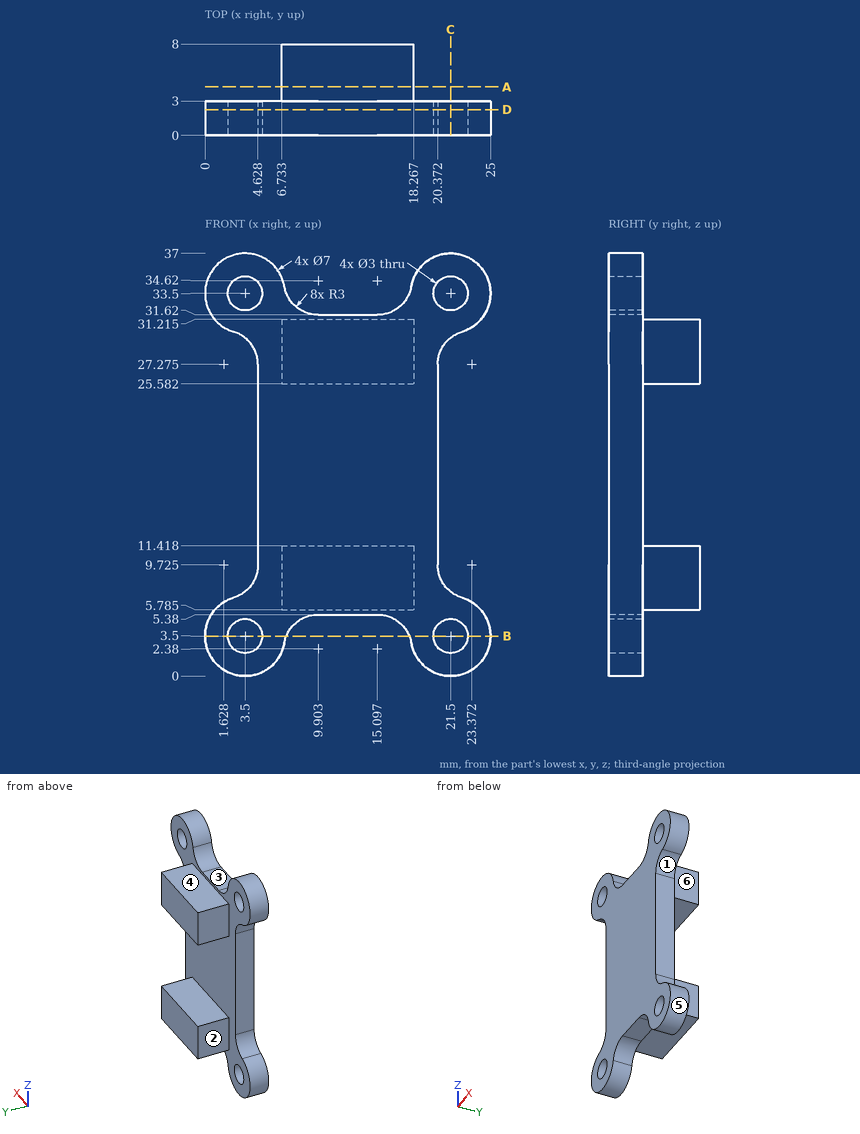
Source: three-view drawing plus pictorial views. Frame: mm from the lowest corner of the part. A direction names the side the tool comes from. Coordinates: 2 decimals unless noted, no trailing zeros. Loops run counter-clockwise (first coordinate to the right, second up) from the corner with the lowest first, then second, coordinate; pieces in that order, holes last. Notation, with made-up numbers: (3.5, 32) -> (42.5, 32) arc R10 cw to (42.5, 45) -> close; hole circle Ø5 at (43, 0). An arc over 180 degrees is marked (long way). Write each question's results on one line, items separated by ' | '. Start each with the question number.
Q1. Section A-A, the plane y = 4.25. Return the cut outline in (x, z) (1 decimal), plus the area to 3 significant figures.
Q2. Pull-direction query (Z, two-part tool) for the marked faces 4, 5 and 6; classes: released by +Z, released by -Z, zero draft, split by the parting line, or undercut.
Q3. Ray query, line 1 (Z direction, x = 7.5, y = 6) (1 decimal); line 2 (X direction, y = 0.95, z = 33.5); line 3 (Z direction, x = 12.5, y = 0.5). Return the intervals inside material, ascending. Write a range as from..to.
Q4. Pin query (flat end, axial travel): pin 1 (1 mm diameter, centred on x = 8, y = 4, fed in from -Z) (1 decimal); pin 2 (4 mm diameter, centred on y = 6, z = 7.5, fed in from +X); pin 3 (0.9 mm diameter, centred on y = 1, z = 21, fed in from +X); pin 4 (12.5 mm diameter, centred on x = 9, z = 24, fed in from +Y). Return the tip coordinate at first contact, or that it passes through.
Q5. Reachability of the marked faces 1, 2 and 3 from +Z, -Z, +X, -X, +Y, -Y: full face, straight path, thin tool, end or side. Return the list, or none.
Q6. Section D-D, the plane y = 2.25. Return the cut outline in (x, z) (1 decimal), plus the area to 3 significant figures.
Q7. Section C-C, the plane x = 21.5. Return the cut outline in (y, z).
Q8. Section B-B, the plane z = 3.5. Return the cut outline in (x, y).
Found:
1) outline: (6.7, 5.8) -> (18.3, 5.8) -> (18.3, 11.4) -> (6.7, 11.4) -> close; (6.7, 25.6) -> (18.3, 25.6) -> (18.3, 31.2) -> (6.7, 31.2) -> close | area: 130 mm2
2) face 4: released by +Z | face 5: undercut | face 6: zero draft
3) line 1: 5.8..11.4, 25.6..31.2 | line 2: 0..2, 5..7.12, 17.88..20, 23..25 | line 3: 5.38..31.62
4) pin 1: z = 5.8 | pin 2: x = 18.27 | pin 3: x = 20.37 | pin 4: y = 8
5) face 1: +X, +Y, -Y | face 2: +Z, -Z, -X, +Y | face 3: +Z, +Y, -Y
6) outline: (2.5, 6.9) arc R3.5 ccw (long way) to (6.9, 2.9) arc R3 cw to (9.9, 5.4) -> (15.1, 5.4) arc R3 cw to (18.1, 2.9) arc R3.5 ccw (long way) to (22.5, 6.9) arc R3 cw to (20.4, 9.7) -> (20.4, 27.3) arc R3 cw to (22.5, 30.1) arc R3.5 ccw (long way) to (18.1, 34.1) arc R3 cw to (15.1, 31.6) -> (9.9, 31.6) arc R3 cw to (6.9, 34.1) arc R3.5 ccw (long way) to (2.5, 30.1) arc R3 cw to (4.6, 27.3) -> (4.6, 9.7) arc R3 cw to start; hole circle Ø3 at (3.5, 3.5); hole circle Ø3 at (3.5, 33.5); hole circle Ø3 at (21.5, 3.5); hole circle Ø3 at (21.5, 33.5) | area: 546 mm2
7) outline: (0, 0) -> (3, 0) -> (3, 2) -> (0, 2) -> close; (0, 5) -> (3, 5) -> (3, 7.38) -> (0, 7.38) -> close; (0, 29.62) -> (3, 29.62) -> (3, 32) -> (0, 32) -> close; (0, 35) -> (3, 35) -> (3, 37) -> (0, 37) -> close
8) outline: (0, 0) -> (2, 0) -> (2, 3) -> (0, 3) -> close; (5, 0) -> (7.12, 0) -> (7.12, 3) -> (5, 3) -> close; (17.88, 0) -> (20, 0) -> (20, 3) -> (17.88, 3) -> close; (23, 0) -> (25, 0) -> (25, 3) -> (23, 3) -> close
